Source: CAD feature listing. Evaluate the final solid. Frame: model axes, mm. Face numbers are marked on the shaded views. A direction names the side the tool comes from. Round coordinates to 2 decimals unless told otherwise and drop trailing zeros. Write each loop counter-clockwise with the first axis right and the second up, starting at its lowest first coordinate (ties: lowest second). Pieces come first, ordered by that corner, then holes. Notation, with made-up numbers: M 62,-6 L 72,-6 A18 ccw 72,0 Z; hole C 64,-12.75 d4. An arc over 180 degrees is marked long. Answer in a Markdown table with one row per item. Add a question column.
Item 1: Contact query for flat-ended pins moving along their axis: pin 1 (0.9 mm diameter, centred on x = 1.65, z = 18.55, fed in from +Y); pin 2 (1.5 mm diameter, centred on x = 2, z = 2.5, fed in from -Y); pin 3 (2 mm diameter, centred on x = -3, z = 3, fed in from +Y); pin 4 (2 mm diameter, centred on x = 0, z = 6.5, fed in from -Y). Output: stop coordinate, or through.
Item 2: Cut plane D-D on y = 0. Return loops of the section in (x, z), and give its area (3 significant figures).
Item 3: Cut plane C-C on x = 0. Give the number of separate pieces and of enclosed holes in the cut face, and give its area (3 significant figures).
Item 4: Cut plane A-A on y = -2. Return loops of the section in (x, z), and give its area (3 significant figures).
Item 5: Mould query, pull axis X, two halves, no side actions, for the marked faces 1, 2, 3 and 4. Classes: released by +X, released by -X, zero draft, split by the parting line, or undercut.
Item 6: Set-up query: the marked faces 5 and 6. Return all of +Z, -Z, +X, -X, +Y, -Y with unobstructed straight access to the full face (end or side cutting, diameter ignored); none if empty.
Item 7: Material intervals for probe 1 along Z at (x, y) = (0, -2.2); probe 2 along Z at (x, y) = (0, -1.75); probe 3 along Y at (x, z) = (1, 5), sorted ascending.
Autodesk Inventor part; units mm, degrees
ref_plane "YZ Plane" through (0, 0, 0) normal (1, 0, 0) x (0, 1, 0)
ref_plane "XZ Plane" through (0, 0, 0) normal (0, 1, 0) x (-1, 0, 0)
sketch "Sketch1" plane through (0, 0, 0) normal (0, 0, 1) x (1, 0, 0)
  line L0 (0, 3.81) -> (1.746, 3.81)
  line L1 (0, 0) -> (0, 7.4896) construction
  line L2 (0, 0) -> (13.1944, 0) construction
  line L3 (0, -3.81) -> (1.746, -3.81)
  arc A0 (1.746, -3.81) -> (1.746, 3.81) centre (0, 0) ccw
  line L4 (0, 3.81) -> (0, -3.81)
  point P0 (-6.8886, 3.81)
  point P1 (6.6767, 3.81)
  point P2 (0, 4.191)
  point P3 (0, 4.191)
  point P4 (-6.8886, -3.81)
  point P5 (6.6767, -3.81)
  point P6 (0, 4.191)
  point P7 (4.191, 0)
  dimension "d1" = 0.381
  dimension "d11" = 4.191
revolve "Revolution1" add sketch "Sketch1" angle 360 about axis through (0, 0, 0) along (0, 1, 0)
sketch "Sketch2" plane through (0, 3.81, 0) normal (0, 1, 0) x (1, 0, 0)
  circle A0 centre (0, 0) radius 1.746
  dimension "d3" = 3.4919
hole "Hole1" at (0, 3.81, 0) direction (0, -1, 0) diameter 3.4798 end through all
ref_plane "Work Plane1" through (0, 0, 4.191) normal (0, 0, 1) x (1, 0, 0)
sketch "Sketch3" plane through (0, 0, 4.191) normal (0, 0, 1) x (1, 0, 0)
  line L0 (-2.159, 2.54) -> (2.159, 2.54)
  line L1 (2.159, 2.54) -> (2.159, -1.27)
  line L2 (2.159, -1.27) -> (-2.159, -1.27)
  line L3 (-2.159, -1.27) -> (-2.159, 2.54)
  line L4 (1.746, 3.81) -> (-1.746, 3.81)
  point P0 (0, 0)
  point P1 (0, 2.54)
  dimension "d13" = 4.318
  dimension "d14" = 3.81
  dimension "d15" = 1.27
extrude "Extrusion1" add sketch "Sketch3" along normal blind 10.16
ref_plane "Work Plane2" through (0, 0, 1.7399) normal (0, 0, 1) x (1, 0, 0)
extrude "Extrusion2" add sketch "Sketch3" against normal up to surface (2.4511 mm away)
sketch "Sketch4" plane through (0, -1.27, 0) normal (0, -1, 0) x (1, 0, 0)
  line L0 (2.159, 2.54) -> (2.159, 14.351)
  line L1 (2.159, 10.541) -> (-2.159, 10.541)
  line L2 (-2.159, 10.541) -> (-2.159, 14.351)
  line L3 (-2.159, 14.351) -> (2.159, 14.351)
  line L4 (2.159, 14.351) -> (2.159, 10.541) construction
  line L5 (-2.159, 14.351) -> (2.159, 14.351)
  circle A0 centre (0, 15.689) radius 0.762
  circle A1 centre (0, 15.689) radius 2.54
  circle A2 centre (1.651, 18.5486) radius 0.762
  circle A3 centre (1.651, 18.5486) radius 2.54
  point P0 (0, 0)
  point P1 (2.159, 14.351)
  point P2 (0, 14.351)
  point P3 (2.159, 14.351)
  point P4 (4.191, 18.5486)
  point P5 (-0.8461, 18.084)
  point P6 (1.27, 17.8887)
  point P7 (2.4971, 16.1537)
  point P8 (-0.889, 18.5486)
  dimension "d22" = 3.81
  dimension "d25" = 1.524
  dimension "d27" = 5.08
  dimension "d30" = 1.524
  dimension "d31" = 5.08
  dimension "d33" = 4.318
  dimension "d34" = 1.27
extrude "Extrusion4" add sketch "Sketch4" along normal blind 1.27
properties part number "Left Arm" material "Phenolic Resin"
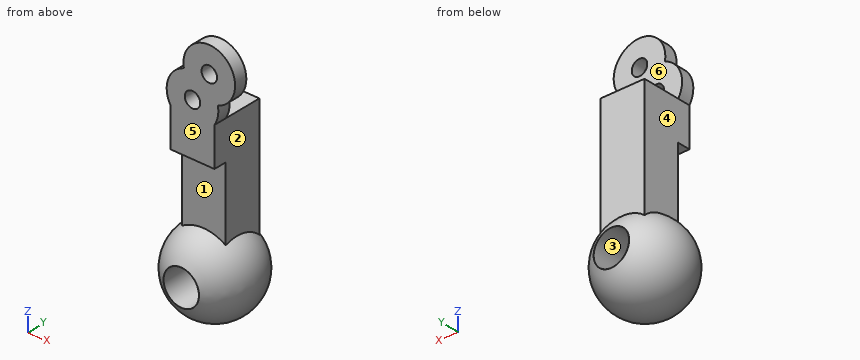
Results below:
| question | item | result |
|---|---|---|
| 1 | pin 1 | through |
| 1 | pin 2 | y = -3.4 |
| 1 | pin 3 | y = 2.66 |
| 1 | pin 4 | y = -1.27 |
| 2 | outline | M -2.16,3.59 A4.19 ccw long 2.16,3.59 L 2.16,14.35 L -2.16,14.35 Z; hole C 0,0 d3.48 |
| 2 | area | 90.4 mm2 |
| 3 | separate pieces | 3 |
| 3 | enclosed holes | 0 |
| 3 | area | 77.0 mm2 |
| 4 | outline | C 0,0 d7.37; M -2.16,10.54 L 2.16,10.54 L 2.16,14.35 A2.54 ccw 2.5,16.15 A2.54 ccw long -0.85,18.08 A2.54 ccw -2.16,14.35 Z; hole C 0,0 d3.48; hole C 0,15.69 d1.52; hole C 1.65,18.55 d1.52 |
| 4 | area | 78.0 mm2 |
| 5 | face 1 | zero draft |
| 5 | face 2 | released by +X |
| 5 | face 3 | undercut |
| 5 | face 4 | released by -X |
| 6 | face 5 | +Z, +X, -X, -Y |
| 6 | face 6 | +Z, +X, -X, +Y |
| 7 | probe 1 | -3.57 to -1.74, 1.74 to 3.57, 10.54 to 14.93, 16.45 to 20.48 |
| 7 | probe 2 | -3.81 to -1.74, 1.74 to 3.81, 10.54 to 14.93, 16.45 to 20.48 |
| 7 | probe 3 | -1.27 to 2.54 |
